The model under review builds one solid part; all positions refer to its coordinate system, in mm. A direction names the side the tool comes from. Coordinates: 2 decimals unless noted, no trailing zeros. Write each loop counter-clockwise with the first axis right and the second up, starting at its lowest first coordinate (ties: lowest second). Pieces come first, ordered by that corner, then holes. Notation, with made-up numbers: (-13.75, 28.5) - (13.25, 28.5) arc R30 cw to (13.25, 59.5) - close; hole circle Ø6 at (51.25, 8). An arc over 180 degrees is marked (long way). Put each result on its own line as item: value.
from build123d import *

# Parameters (mm, degrees)
FRAME_DEPTH         = 10
SKETCH13_R          = 3.5
CUT_EXTRUDE7_DEPTH  = 67.66634461
FILLET4_R           = 1
SKETCH14_W          = 5
SKETCH14_H          = 5
CUT_EXTRUDE8_DEPTH  = 81.777611378
FILLET5_R           = 2
CUT_EXTRUDE9_DEPTH  = 5
CHAMFER1_SIZE       = 1
FILLET6_R           = 2
FILLET7_R           = 1
CUT_EXTRUDE11_REACH = 59.656
SKETCH18_R          = 2.5
CUT_EXTRUDE12_REACH = 83.008
SKETCH19_R          = 2.5


with BuildPart() as part:
    # Sketch1 → Frame (new body)
    with BuildSketch(Plane.XY):
        Polygon((-8, 62.65), (49, 62.65), (49, 52.65), (48, 52.65), (48, 60.65), (42, 60.65), (42, 6.5), (44.7, 2), (48, 2), (49, 2.703504174), (50, 2.703504174), (50, -0.296495826), (37, -0.296495826), (-8, 42.65), (-18, 42.65), (-18, 62.65), align=None)
        Polygon((-8, 44.65), (-8, 60.65), (38.585786438, 60.65), (7.695355997, 29.759569559), align=None, mode=Mode.SUBTRACT)
        Polygon((40, 59.235786438), (40, 1.703504174), (37.268035971, 1.703504174), (9.146787391, 28.382573828), align=None, mode=Mode.SUBTRACT)
    extrude(amount=FRAME_DEPTH)

    # Sketch13 → Cut-Extrude7 (cut, through all)
    with BuildSketch(Plane.XZ.offset(-42.65)):
        with Locations(Location((-13, 5, 0), (0, 0, 270))):
            Circle(SKETCH13_R)
    extrude(amount=-CUT_EXTRUDE7_DEPTH, mode=Mode.SUBTRACT)

    # Fillet4
    fillet4_edges = [part.edges().sort_by_distance(p)[0] for p in [
        (-13, 62.65, 8.5),
        (-13, 42.65, 8.5),
    ]]
    fillet(fillet4_edges, radius=FILLET4_R)

    # Sketch14 → Cut-Extrude8 (cut, through all)
    with BuildSketch(Plane.XY.offset(10)):
        with Locations((-15.5, 52.15)):
            Rectangle(SKETCH14_W, SKETCH14_H)
    extrude(amount=-CUT_EXTRUDE8_DEPTH, mode=Mode.SUBTRACT)

    # Fillet5
    fillet5_edges = [part.edges().sort_by_distance(p)[0] for p in [
        (-18, 58.65, 0),
        (-18, 58.65, 10),
        (-18, 46.15, 0),
        (-18, 46.15, 10),
    ]]
    fillet(fillet5_edges, radius=FILLET5_R)

    # Sketch15 → Cut-Extrude9 (cut)
    with BuildSketch(Plane(origin=(0, 49.65, 0), x_dir=(1, 0, 0), z_dir=(0, 1, 0))):
        Polygon((-10, 0), (-8, -2), (-8, 0), align=None)
        Polygon((-10, -10), (-8, -8), (-8, -10), align=None)
    extrude(amount=CUT_EXTRUDE9_DEPTH, mode=Mode.SUBTRACT)

    # Chamfer1
    chamfer1_edges = [part.edges().sort_by_distance(p)[0] for p in [
        (-13, 52.15, 0),
        (-13, 52.15, 10),
    ]]
    chamfer(chamfer1_edges, length=CHAMFER1_SIZE)

    # Fillet6
    # the kernel refuses this fillet: 2 mm, written as the material it adds along each edge
    with BuildSketch(Plane(origin=(-8, 60.65, 0), x_dir=(0, -1, 0), z_dir=(0, 0, 1)), Plane(origin=(40, 1.703504174, 0), x_dir=(0, 1, 0), z_dir=(0, 0, 1))) as fillet6_piece_1:
        with BuildLine():
            CenterArc((FILLET6_R, FILLET6_R), FILLET6_R, 180, 90)
            Line((0, FILLET6_R), (0, 0))
            Line((0, 0), (FILLET6_R, 0))
        make_face()
    extrude(amount=10)
    with BuildSketch(Plane(origin=(37.268035971, 1.703504174, 0), x_dir=(1, 0, 0), z_dir=(0, 0, 1))) as fillet6_piece_2:
        with BuildLine():
            CenterArc((FILLET6_R * 0.398883640348, FILLET6_R), FILLET6_R, 226.507503973, 43.492496027)
            Line((-FILLET6_R * 0.289375927855, FILLET6_R * 0.274535482069), (0, 0))
            Line((0, 0), (FILLET6_R * 0.398883640348, 0))
        make_face()
    extrude(amount=10)
    with BuildSketch(Plane(origin=(-8, 44.65, 0), x_dir=(0, 1, 0), z_dir=(0, 0, 1))) as fillet6_piece_3:
        with BuildLine():
            CenterArc((FILLET6_R * 0.429711480151, -FILLET6_R), FILLET6_R, 90, 46.507503973)
            Line((-FILLET6_R * 0.29575303778, -FILLET6_R * 0.311740431797), (0, 0))
            Line((0, 0), (FILLET6_R * 0.429711480151, 0))
        make_face()
    extrude(amount=10)
    with BuildSketch(Plane(origin=(9.146787391, 28.382573828, 0), x_dir=(0.7254645179309741, -0.6882595682031448, 0), z_dir=(0, 0, 1))) as fillet6_piece_4:
        with BuildLine():
            CenterArc((FILLET6_R * 1.02666321267, FILLET6_R), FILLET6_R, 178.492496027, 91.507503973)
            Line((FILLET6_R * 0.0270093246389, FILLET6_R * 1.02630787225), (0, 0))
            Line((0, 0), (FILLET6_R * 1.02666321267, 0))
        make_face()
    extrude(amount=10)
    with BuildSketch(Plane(origin=(7.695355997, 29.759569559, 0), x_dir=(0.7071067811865478, 0.7071067811865474, 0), z_dir=(0, 0, 1))) as fillet6_piece_5:
        with BuildLine():
            CenterArc((FILLET6_R * 0.974029250934, FILLET6_R), FILLET6_R, 181.507503973, 88.492496027)
            Line((-FILLET6_R * 0.0256246370977, FILLET6_R * 0.973692127754), (0, 0))
            Line((0, 0), (FILLET6_R * 0.974029250934, 0))
        make_face()
    extrude(amount=10)

    # Fillet7
    fillet7_edges = [part.edges().sort_by_distance(p)[0] for p in [
        (38.585786438, 60.65, 5),
        (40, 59.235786438, 5),
    ]]
    fillet(fillet7_edges, radius=FILLET7_R)

    # Sketch18 → Cut-Extrude11 (cut, up to next)
    with BuildSketch(Plane(origin=(17.488453969, 18.324671512, 0), x_dir=(0.7234201739583832, -0.6904080329124386, 0), z_dir=(-0.6904080329124386, -0.7234201739583832, 0)), mode=Mode.PRIVATE) as cut_extrude11_sk1:
        with Locations((-26.968990252, 5)):
            Circle(SKETCH18_R)
    cut_extrude11_tool1 = extrude(cut_extrude11_sk1.sketch, amount=-CUT_EXTRUDE11_REACH, mode=Mode.PRIVATE) & part.part
    # Sketch18 → Cut-Extrude11 (cut, up to next)
    with BuildSketch(Plane(origin=(17.488453969, 18.324671512, 0), x_dir=(0.7234201739583832, -0.6904080329124386, 0), z_dir=(-0.6904080329124386, -0.7234201739583832, 0)), mode=Mode.PRIVATE) as cut_extrude11_sk2:
        with Locations((-17.968990252, 5)):
            Circle(SKETCH18_R)
    cut_extrude11_tool2 = extrude(cut_extrude11_sk2.sketch, amount=-CUT_EXTRUDE11_REACH, mode=Mode.PRIVATE) & part.part
    # Sketch18 → Cut-Extrude11 (cut, up to next)
    with BuildSketch(Plane(origin=(17.488453969, 18.324671512, 0), x_dir=(0.7234201739583832, -0.6904080329124386, 0), z_dir=(-0.6904080329124386, -0.7234201739583832, 0)), mode=Mode.PRIVATE) as cut_extrude11_sk3:
        with Locations((-8.968990252, 5)):
            Circle(SKETCH18_R)
    cut_extrude11_tool3 = extrude(cut_extrude11_sk3.sketch, amount=-CUT_EXTRUDE11_REACH, mode=Mode.PRIVATE) & part.part
    # Sketch18 → Cut-Extrude11 (cut, up to next)
    with BuildSketch(Plane(origin=(17.488453969, 18.324671512, 0), x_dir=(0.7234201739583832, -0.6904080329124386, 0), z_dir=(-0.6904080329124386, -0.7234201739583832, 0)), mode=Mode.PRIVATE) as cut_extrude11_sk4:
        with Locations((0.031009748, 5)):
            Circle(SKETCH18_R)
    cut_extrude11_tool4 = extrude(cut_extrude11_sk4.sketch, amount=-CUT_EXTRUDE11_REACH, mode=Mode.PRIVATE) & part.part
    # Sketch18 → Cut-Extrude11 (cut, up to next)
    with BuildSketch(Plane(origin=(17.488453969, 18.324671512, 0), x_dir=(0.7234201739583832, -0.6904080329124386, 0), z_dir=(-0.6904080329124386, -0.7234201739583832, 0)), mode=Mode.PRIVATE) as cut_extrude11_sk5:
        with Locations((9.031009748, 5)):
            Circle(SKETCH18_R)
    cut_extrude11_tool5 = extrude(cut_extrude11_sk5.sketch, amount=-CUT_EXTRUDE11_REACH, mode=Mode.PRIVATE) & part.part
    # Sketch18 → Cut-Extrude11 (cut, up to next)
    with BuildSketch(Plane(origin=(17.488453969, 18.324671512, 0), x_dir=(0.7234201739583832, -0.6904080329124386, 0), z_dir=(-0.6904080329124386, -0.7234201739583832, 0)), mode=Mode.PRIVATE) as cut_extrude11_sk6:
        with Locations((18.031009748, 5)):
            Circle(SKETCH18_R)
    cut_extrude11_tool6 = extrude(cut_extrude11_sk6.sketch, amount=-CUT_EXTRUDE11_REACH, mode=Mode.PRIVATE) & part.part
    add(cut_extrude11_tool1.solids().sort_by_distance((-2.021458, 36.944279, 5))[0], mode=Mode.SUBTRACT)
    add(cut_extrude11_tool2.solids().sort_by_distance((4.489324, 30.730607, 5))[0], mode=Mode.SUBTRACT)
    add(cut_extrude11_tool3.solids().sort_by_distance((11.000105, 24.516934, 5))[0], mode=Mode.SUBTRACT)
    add(cut_extrude11_tool4.solids().sort_by_distance((17.510887, 18.303262, 5))[0], mode=Mode.SUBTRACT)
    add(cut_extrude11_tool5.solids().sort_by_distance((24.021669, 12.08959, 5))[0], mode=Mode.SUBTRACT)
    add(cut_extrude11_tool6.solids().sort_by_distance((30.53245, 5.875918, 5))[0], mode=Mode.SUBTRACT)

    # Sketch19 → Cut-Extrude12 (cut, up to next)
    with BuildSketch(Plane(origin=(0, 62.65, 0), x_dir=(1, 0, 0), z_dir=(0, 1, 0)), mode=Mode.PRIVATE) as cut_extrude12_sk1:
        with Locations(Location((-1.5, -5, 0), (0, 0, 180))):
            Circle(SKETCH19_R)
    cut_extrude12_tool1 = extrude(cut_extrude12_sk1.sketch, amount=-CUT_EXTRUDE12_REACH, mode=Mode.PRIVATE) & part.part
    # Sketch19 → Cut-Extrude12 (cut, up to next)
    with BuildSketch(Plane(origin=(0, 62.65, 0), x_dir=(1, 0, 0), z_dir=(0, 1, 0)), mode=Mode.PRIVATE) as cut_extrude12_sk2:
        with Locations(Location((6.5, -5, 0), (0, 0, 180))):
            Circle(SKETCH19_R)
    cut_extrude12_tool2 = extrude(cut_extrude12_sk2.sketch, amount=-CUT_EXTRUDE12_REACH, mode=Mode.PRIVATE) & part.part
    # Sketch19 → Cut-Extrude12 (cut, up to next)
    with BuildSketch(Plane(origin=(0, 62.65, 0), x_dir=(1, 0, 0), z_dir=(0, 1, 0)), mode=Mode.PRIVATE) as cut_extrude12_sk3:
        with Locations(Location((14.5, -5, 0), (0, 0, 180))):
            Circle(SKETCH19_R)
    cut_extrude12_tool3 = extrude(cut_extrude12_sk3.sketch, amount=-CUT_EXTRUDE12_REACH, mode=Mode.PRIVATE) & part.part
    # Sketch19 → Cut-Extrude12 (cut, up to next)
    with BuildSketch(Plane(origin=(0, 62.65, 0), x_dir=(1, 0, 0), z_dir=(0, 1, 0)), mode=Mode.PRIVATE) as cut_extrude12_sk4:
        with Locations(Location((22.5, -5, 0), (0, 0, 180))):
            Circle(SKETCH19_R)
    cut_extrude12_tool4 = extrude(cut_extrude12_sk4.sketch, amount=-CUT_EXTRUDE12_REACH, mode=Mode.PRIVATE) & part.part
    # Sketch19 → Cut-Extrude12 (cut, up to next)
    with BuildSketch(Plane(origin=(0, 62.65, 0), x_dir=(1, 0, 0), z_dir=(0, 1, 0)), mode=Mode.PRIVATE) as cut_extrude12_sk5:
        with Locations(Location((30.5, -5, 0), (0, 0, 180))):
            Circle(SKETCH19_R)
    cut_extrude12_tool5 = extrude(cut_extrude12_sk5.sketch, amount=-CUT_EXTRUDE12_REACH, mode=Mode.PRIVATE) & part.part
    add(cut_extrude12_tool1.solids().sort_by_distance((-1.5, 62.65, 5))[0], mode=Mode.SUBTRACT)
    add(cut_extrude12_tool2.solids().sort_by_distance((6.5, 62.65, 5))[0], mode=Mode.SUBTRACT)
    add(cut_extrude12_tool3.solids().sort_by_distance((14.5, 62.65, 5))[0], mode=Mode.SUBTRACT)
    add(cut_extrude12_tool4.solids().sort_by_distance((22.5, 62.65, 5))[0], mode=Mode.SUBTRACT)
    add(cut_extrude12_tool5.solids().sort_by_distance((30.5, 62.65, 5))[0], mode=Mode.SUBTRACT)


solid = part.part
1. For pin 1 Ø4 at (y, z) = (26, 2.5) entering from +X; pin 2 Ø8 at (x, y) = (-7.5, 52.5) entering from +Z; pin 3 Ø3 at (y, z) = (36, 6) entering from -X; pin 4 Ø5 at (x, z) = (-13.5, 7) entering from -Y, all flat-tipped, find the tip position at first contact; note any pin that passes through.
Determined:
pin 1: stops at x = 42
pin 2: stops at z = 10
pin 3: stops at x = -1.55
pin 4: stops at y = 42.65
2. The part is to be moulded in two halves that separate along Y. For faces 6 (the cylindrical face through (-17.4, 58.71, 9.43)), 7 (the flat face through (23.17, 45.235, 4.93)), 8 (the flat face through (-8.5, 42.65, 3.8)), say which applies: +Y half, -Y half, draft (parallel to the pull), parting line (faces both ways), or undercut.
Determined:
face 6: draft
face 7: undercut
face 8: -Y half
3. Machinability: for faces 1 (the flat face through (-8.5, 54.65, 9.4)), 2 (the cylindrical face through (-1.17, 61.66, 7.48)), 3 (the flat face through (49, 58, 5)), 4 (the flat face through (-8.6, 49.65, 0.5)), 5 (the flat face through (48, 57, 5)), which of the approach directions +Z, -Z, +X, -X, +Y, -Y give a long, thin tool a straight path to every point of the face, cutting with its end or side? Answer none if there is none.
Determined:
face 1: +Z
face 2: +Y
face 3: +Z, -Z, +X, +Y
face 4: -Z
face 5: +Z, -Z
4. To check wall thickness, follow probe 1 along Z at (x, y) = (6.5, 61.95); probe 2 along X at (y, z) = (37, 8.75); probe 3 along X at (y, z) = (60, 1.25). State the ranges of each line that lie inside material, in increasing order.
Determined:
probe 1: z = 0 to 2.5, 7.5 to 10
probe 2: x = -2.08 to 0.06, 14.94 to 17.76, 40 to 42
probe 3: x = -17.85 to -7.48, 37.11 to 42, 48 to 49
5. Consider section A-A on y = 47. State the section outline as (x, z) points.
Determined:
outline: (-18, 2) arc R2 ccw to (-16, 0) - (-8, 0) - (-8, 10) - (-16, 10) arc R2 ccw to (-18, 8) - close; (24.94, 0) - (27.76, 0) - (27.76, 10) - (24.94, 10) - close; (40, 0) - (42, 0) - (42, 10) - (40, 10) - close; hole circle Ø7 at (-13, 5)
6. Consider section B-B on z = 5. Give the number of separate pieces and of enclosed holes in the cut face, plus the area to 3 significant figures.
Determined:
separate pieces: 12
enclosed holes: 0
area: 421 mm^2
